Can you work these out from the model? Positions are in its coordinate system, mm. Coordinates: 2 decimals unless noted, no trailing zeros. Order: outer loops, then holes, each group sorted by start corner. A loop starts at its lowest first (then second) coordinate and runs counter-clockwise, first axis right, second up.
```python
from build123d import *

# Parameters (mm, degrees)
BOSS_EXTRUDE1_DEPTH = 2
SKETCH3_W           = 2.352038348
SKETCH3_H           = 29.381645189
CUT_EXTRUDE1_DEPTH  = 10
BOSS_EXTRUDE6_DEPTH = 2
BOSS_EXTRUDE9_DEPTH = 2


with BuildPart() as part:
    # Sketch1 → Boss-Extrude1 (new body)
    with BuildSketch(Plane(origin=(0, 0, 0), x_dir=(1, 0, 0), z_dir=(0, 1, 0))):
        with BuildLine():
            Line((2.5, -24.892218109), (2.5, 17.168276032))
            ThreePointArc((2.5, 17.168276032), (-0.157753681, 18.055867427), (-2.504670814, 16.525033312))
            Line((-2.504670814, 16.525033312), (-2.504670814, -24.882267467))
            ThreePointArc((-2.504670814, -24.882267467), (-0.005496175, -26.4769499), (2.5, -24.892218109))
        make_face()
    extrude(amount=BOSS_EXTRUDE1_DEPTH)

    # Sketch3 → Cut-Extrude1 (cut)
    with BuildSketch(Plane(origin=(0, 0, 0), x_dir=(-1, 0, 0), z_dir=(0, -1, 0))):
        with Locations((0.225062248, -3.353285415)):
            Rectangle(SKETCH3_W, SKETCH3_H)
    extrude(amount=-CUT_EXTRUDE1_DEPTH, mode=Mode.SUBTRACT)

    # Sketch8 → Boss-Extrude6 (add)
    with BuildSketch(Plane(origin=(0, 0, 0), x_dir=(-1, 0, 0), z_dir=(0, -1, 0))):
        Polygon((0.354887885, 16.216439576), (-1.169599114, 15.336276597), (-1.169599114, 13.575950638), (0.354887885, 12.695787659), (1.879374884, 13.575950638), (1.879374884, 15.336276597), align=None)
    extrude(amount=BOSS_EXTRUDE6_DEPTH)

    # Sketch9 → Boss-Extrude9 (add)
    with BuildSketch(Plane(origin=(0, 0, 0), x_dir=(-1, 0, 0), z_dir=(0, -1, 0))):
        Polygon((-1.616477648, 0.618051223), (-0.699382455, -0.970404247), (1.13480793, -0.970404247), (2.051903123, 0.618051223), (1.13480793, 2.206506692), (-0.699382455, 2.206506692), align=None)
    extrude(amount=BOSS_EXTRUDE9_DEPTH)


solid = part.part
```
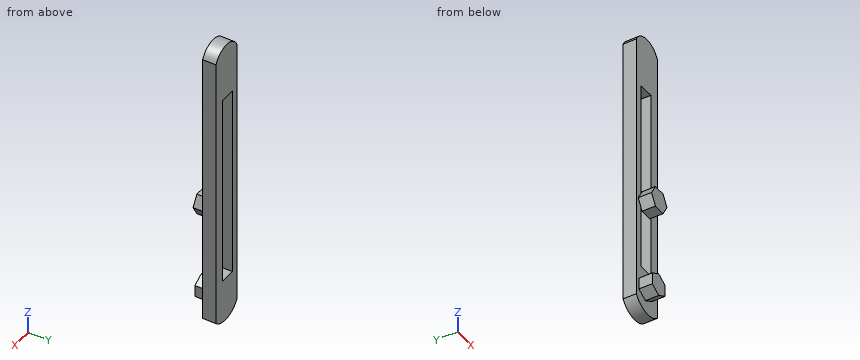
1. Please list where these lines run through material, in increasing order: probe 1 along X at (y, z) = (0.25, -3.5); probe 2 along Y at (x, z) = (-1.55, 9); probe 3 along Z at (x, y) = (-0.4, -1.25).
Completed:
probe 1: x = -2.5 to -1.4, 0.95 to 2.5
probe 2: y = 0 to 2
probe 3: z = -16.19 to -12.72, -2.21 to 0.97
2. I'm going to push flat-ended pins straight in: pin 1 (0.9 mm diameter, centred on y = -1.5, z = -14.5, fed in from -X); pin 2 (0.7 mm diameter, centred on x = -0.5, z = -1, fed in from +Y); pin 3 (0.5 mm diameter, centred on y = -0.5, z = -14.5, fed in from +X); pin 4 (1 mm diameter, centred on y = -1, z = 20.5, fed in from +X). Where does each tip first touch, or does it pass through?
Completed:
pin 1: stops at x = -1.88
pin 2: stops at y = 0
pin 3: stops at x = 1.17
pin 4: passes through
3. Imagine slicing it at B-B on z = -6. Please give me the cut outline in (x, y).
Completed:
outline: (-2.5, 0) - (-1.4, 0) - (-1.4, 2) - (-2.5, 2) - close; (0.95, 0) - (2.5, 0) - (2.5, 2) - (0.95, 2) - close
4. Imagine slicing it at D-D on z = 22. Please give me the cut outline in (x, y), then the cut area to 3 significant figures.
Completed:
outline: (-2.5, 0) - (2.5, 0) - (2.5, 2) - (-2.5, 2) - close
area: 10.0 mm2
5. Imagine slicing it at C-C on y = 1. Please give me the cut outline in (x, z), then the cut area to 3 significant figures.
Completed:
outline: (-2.5, -16.53) arc R3.22 ccw to (2.5, -17.17) - (2.5, 24.89) arc R2.76 ccw to (-2.5, 24.88) - close; hole (-1.4, -11.34) - (0.95, -11.34) - (0.95, 18.04) - (-1.4, 18.04) - close
area: 150 mm2
6. Imagine slicing it at A-A on y = -0.8. Please give me the cut outline in (x, z), then the cut area to 3 significant figures.
Completed:
outline: (-2.05, -0.62) - (-1.13, -2.21) - (0.7, -2.21) - (1.62, -0.62) - (0.7, 0.97) - (-1.13, 0.97) - close; (-1.88, -15.34) - (-0.35, -16.22) - (1.17, -15.34) - (1.17, -13.58) - (-0.35, -12.7) - (-1.88, -13.58) - close
area: 16.8 mm2
